For this review, take the finished solid that the model builds, in its own axes (mm). A direction names the side the tool comes from. Give positions to 0.01 mm unless a question says otherwise; leave off trailing zeros. Loops run counter-clockwise (first coordinate to the right, second up) from the corner with the lowest first, then second, coordinate; pieces in that order, holes last. Notation, with made-up numbers: (59, 2.5) - (74, 2.5) arc R18 cw to (74, 9.5) - close; hole circle Ø3 at (0.25, 31.5). An arc over 180 degrees is marked (long way). Put each result on its own line as item: value.
Autodesk Inventor part; units mm, degrees
ref_plane "YZ Plane" through (0, 0, 0) normal (1, 0, 0) x (0, 1, 0)
ref_plane "XZ Plane" through (0, 0, 0) normal (0, 1, 0) x (-1, 0, 0)
ref_plane "XY Plane" through (0, 0, 0) normal (0, 0, 1) x (1, 0, 0)
ref_plane "Work Plane1" through (0, 0, 0) normal (0, 0, 1) x (1, 0, 0)
sketch "Sketch1" plane through (0, 0, 0) normal (0, 0, 1) x (1, 0, 0)
  arc A0 (-3.651, 13.5937) -> (-4.7619, 15.391) centre (-4.2064, 14.4923) ccw
  arc A1 (-3.651, 13.5937) -> (-6.4477, 10.2643) centre (0, 7.6875) ccw
  arc A2 (-8.4097, 11.0483) -> (-6.4477, 10.2643) centre (-7.4287, 10.6563) ccw
  arc A3 (-4.7619, 15.391) -> (-8.4097, 11.0483) centre (0, 7.6875) ccw
  arc A4 (6.4477, 10.2643) -> (8.4097, 11.0483) centre (7.4287, 10.6563) ccw
  arc A5 (6.4477, 10.2643) -> (3.651, 13.5937) centre (0, 7.6875) ccw
  arc A6 (4.7619, 15.391) -> (3.651, 13.5937) centre (4.2064, 14.4923) ccw
  arc A7 (8.4097, 11.0483) -> (4.7619, 15.391) centre (0, 7.6875) ccw
  arc A8 (-6.4563, 5.1322) -> (-8.4209, 4.3547) centre (-7.4386, 4.7434) ccw
  arc A9 (-6.4563, 5.1322) -> (-3.651, 1.7813) centre (0, 7.6875) ccw
  arc A10 (-4.7619, -0.016) -> (-3.651, 1.7813) centre (-4.2064, 0.8827) ccw
  arc A11 (-8.4209, 4.3547) -> (-4.7619, -0.016) centre (0, 7.6875) ccw
  arc A12 (3.651, 1.7813) -> (4.7619, -0.016) centre (4.2064, 0.8827) ccw
  arc A13 (3.651, 1.7813) -> (6.4563, 5.1322) centre (0, 7.6875) ccw
  arc A14 (8.4209, 4.3547) -> (6.4563, 5.1322) centre (7.4386, 4.7434) ccw
  arc A15 (4.7619, -0.016) -> (8.4209, 4.3547) centre (0, 7.6875) ccw
  circle A16 centre (10.65, 7.6999) radius 1.15
  circle A17 centre (0, 15.6875) radius 1.0564
  circle A18 centre (0, -0.3125) radius 1.0564
  circle A19 centre (0, 7.6875) radius 5
  circle A20 centre (0, 7.6875) radius 13.7
  line L0 (-116.625, -11.1875) -> (15.375, -11.1875)
  line L1 (15.375, -11.1875) -> (15.375, -7.6875)
  line L2 (-116.625, -7.6875) -> (15.375, -7.6875)
  line L3 (-116.625, -11.1875) -> (-116.625, -7.6875)
  line L4 (15.375, -7.6875) -> (-15.375, -7.6875)
  line L5 (-15.375, -7.6875) -> (-15.375, 22.3125)
  line L6 (-15.375, 22.3125) -> (15.375, 22.3125)
  line L7 (15.375, 22.3125) -> (15.375, -7.6875)
  circle A21 centre (0, 7.6875) radius 14.375
  circle A22 centre (0, 7.6875) radius 5.2
  arc A23 (-3.4406, 13.2535) -> (-4.9722, 15.7312) centre (-4.2064, 14.4923) ccw
  arc A24 (-3.4406, 13.2535) -> (-6.0763, 10.1158) centre (0, 7.6875) ccw
  arc A25 (-8.7812, 11.1968) -> (-6.0763, 10.1158) centre (-7.4287, 10.6563) ccw
  arc A26 (-4.9722, 15.7312) -> (-8.7812, 11.1968) centre (0, 7.6875) ccw
  arc A27 (4.9722, 15.7312) -> (3.4406, 13.2535) centre (4.2064, 14.4923) ccw
  arc A28 (6.0763, 10.1158) -> (3.4406, 13.2535) centre (0, 7.6875) ccw
  arc A29 (6.0763, 10.1158) -> (8.7812, 11.1968) centre (7.4287, 10.6563) ccw
  arc A30 (8.7812, 11.1968) -> (4.9722, 15.7312) centre (0, 7.6875) ccw
  arc A31 (3.4406, 2.1215) -> (6.0844, 5.2794) centre (0, 7.6875) ccw
  arc A32 (3.4406, 2.1215) -> (4.9722, -0.3562) centre (4.2064, 0.8827) ccw
  arc A33 (4.9722, -0.3562) -> (8.7928, 4.2075) centre (0, 7.6875) ccw
  arc A34 (8.7928, 4.2075) -> (6.0844, 5.2794) centre (7.4386, 4.7434) ccw
  arc A35 (-6.0844, 5.2794) -> (-8.7928, 4.2075) centre (-7.4386, 4.7434) ccw
  arc A36 (-6.0844, 5.2794) -> (-3.4406, 2.1215) centre (0, 7.6875) ccw
  arc A37 (-4.9722, -0.3562) -> (-3.4406, 2.1215) centre (-4.2064, 0.8827) ccw
  arc A38 (-8.7928, 4.2075) -> (-4.9722, -0.3562) centre (0, 7.6875) ccw
  circle A39 centre (10.65, 7.6999) radius 1.55
  point P0 (0, 0)
  dimension "d0" = 30
  dimension "d1" = 15.375
  dimension "d2" = 15.375
  dimension "d3" = 0.2
  dimension "d4" = 0.4
  dimension "d5" = 0.4
  dimension "d6" = 0.4
  dimension "d7" = 0.4
  dimension "d8" = 0.4
extrude "Extrusion1" add sketch "Sketch1" along normal blind 1 contours A20 | L2 L5 L6 L7 | A21
sketch "Sketch2" plane through (0, 0, 1) normal (0, 0, 1) x (1, 0, 0)
  line L0 (15.375, 22.3125) -> (-15.375, 22.3125)
  line L1 (-15.375, 22.3125) -> (-15.375, -7.6875)
  line L2 (-15.375, -7.6875) -> (15.375, -7.6875)
  line L3 (15.375, -7.6875) -> (15.375, 22.3125)
  circle A0 centre (0, 15.6875) radius 1.0564
  circle A1 centre (0, -0.3125) radius 1.0564
  circle A2 centre (0, 7.6875) radius 5.2
  arc A3 (-3.4406, 13.2535) -> (-6.0763, 10.1158) centre (0, 7.6875) ccw
  arc A4 (-8.7812, 11.1968) -> (-6.0763, 10.1158) centre (-7.4287, 10.6563) ccw
  arc A5 (-4.9722, 15.7312) -> (-8.7812, 11.1968) centre (0, 7.6875) ccw
  arc A6 (-3.4406, 13.2535) -> (-4.9722, 15.7312) centre (-4.2064, 14.4923) ccw
  arc A7 (6.0763, 10.1158) -> (3.4406, 13.2535) centre (0, 7.6875) ccw
  arc A8 (4.9722, 15.7312) -> (3.4406, 13.2535) centre (4.2064, 14.4923) ccw
  arc A9 (8.7812, 11.1968) -> (4.9722, 15.7312) centre (0, 7.6875) ccw
  arc A10 (6.0763, 10.1158) -> (8.7812, 11.1968) centre (7.4287, 10.6563) ccw
  arc A11 (3.4406, 2.1215) -> (4.9722, -0.3562) centre (4.2064, 0.8827) ccw
  arc A12 (3.4406, 2.1215) -> (6.0844, 5.2794) centre (0, 7.6875) ccw
  arc A13 (8.7928, 4.2075) -> (6.0844, 5.2794) centre (7.4386, 4.7434) ccw
  arc A14 (4.9722, -0.3562) -> (8.7928, 4.2075) centre (0, 7.6875) ccw
  arc A15 (-6.0844, 5.2794) -> (-3.4406, 2.1215) centre (0, 7.6875) ccw
  arc A16 (-4.9722, -0.3562) -> (-3.4406, 2.1215) centre (-4.2064, 0.8827) ccw
  arc A17 (-8.7928, 4.2075) -> (-4.9722, -0.3562) centre (0, 7.6875) ccw
  arc A18 (-6.0844, 5.2794) -> (-8.7928, 4.2075) centre (-7.4386, 4.7434) ccw
  circle A19 centre (10.65, 7.6999) radius 1.55
  arc A20 (4.9722, 15.7312) -> (3.4406, 13.2535) centre (4.2064, 14.4923) ccw
  line L4 (4.2064, 15.9488) -> (15.375, 15.9488)
  line L5 (15.375, -7.6875) -> (15.375, 22.3125)
  line L6 (4.2064, -0.5738) -> (15.375, -0.5738)
  arc A21 (6.0763, 10.1158) -> (8.7812, 11.1968) centre (7.4287, 10.6563) ccw
  line L7 (6.0763, 10.1158) -> (6.0844, 5.2794)
  point P0 (0, 0)
extrude "Extrusion2" add sketch "Sketch2" along normal blind 1.5 contours L3 L4 A8 A7 L7 A12 A11 L6 L2 L1 L0
sketch "Sketch3" plane through (0, 0, 2.5) normal (0, 0, 1) x (1, 0, 0)
  line L0 (15.375, -7.6875) -> (15.375, -0.5738)
  line L1 (15.375, -0.5738) -> (4.2064, -0.5738)
  arc A0 (3.4406, 2.1215) -> (4.2064, -0.5738) centre (4.2064, 0.8827) ccw
  arc A1 (3.4406, 2.1215) -> (6.0844, 5.2794) centre (0, 7.6875) ccw
  line L2 (6.0844, 5.2794) -> (6.0763, 10.1158)
  arc A2 (6.0763, 10.1158) -> (3.4406, 13.2535) centre (0, 7.6875) ccw
  arc A3 (4.2064, 15.9488) -> (3.4406, 13.2535) centre (4.2064, 14.4923) ccw
  line L3 (4.2064, 15.9488) -> (15.375, 15.9488)
  line L4 (15.375, 15.9488) -> (15.375, 22.3125)
  line L5 (15.375, 22.3125) -> (-15.375, 22.3125)
  line L6 (-15.375, 22.3125) -> (-15.375, -7.6875)
  line L7 (-15.375, -7.6875) -> (15.375, -7.6875)
  circle A4 centre (0, 15.6875) radius 1.0564
  circle A5 centre (0, -0.3125) radius 1.0564
  arc A6 (-6.0844, 5.2794) -> (-8.7928, 4.2075) centre (-7.4386, 4.7434) ccw
  arc A7 (-6.0844, 5.2794) -> (-3.4406, 2.1215) centre (0, 7.6875) ccw
  arc A8 (-4.9722, -0.3562) -> (-3.4406, 2.1215) centre (-4.2064, 0.8827) ccw
  arc A9 (-8.7928, 4.2075) -> (-4.9722, -0.3562) centre (0, 7.6875) ccw
  arc A10 (-3.4406, 13.2535) -> (-4.9722, 15.7312) centre (-4.2064, 14.4923) ccw
  arc A11 (-3.4406, 13.2535) -> (-6.0763, 10.1158) centre (0, 7.6875) ccw
  arc A12 (-8.7812, 11.1968) -> (-6.0763, 10.1158) centre (-7.4287, 10.6563) ccw
  arc A13 (-4.9722, 15.7312) -> (-8.7812, 11.1968) centre (0, 7.6875) ccw
  circle A14 centre (0, 7.6875) radius 5.2
  circle A15 centre (0, 15.6875) radius 2.65
  circle A16 centre (0, -0.3125) radius 1.0564
  circle A17 centre (0, -0.3125) radius 2.65
  arc A18 (-2.4425, 10.6818) -> (-4.3563, 11.5819) centre (-5.3868, 6.906) ccw
  arc A19 (-4.3563, 11.5819) -> (-4.9119, 10.8525) centre (0, 7.6875) ccw
  arc A20 (-4.9119, 10.8525) -> (-3.5356, 9.2466) centre (-0.678, 13.0883) ccw
  arc A21 (-3.5356, 9.2466) -> (-3.736, 8.6743) centre (0, 7.6875) ccw
  arc A22 (-3.736, 8.6743) -> (-5.8134, 8.2775) centre (-3.8987, 3.889) ccw
  arc A23 (-5.8134, 8.2775) -> (-5.8341, 7.3609) centre (0, 7.6875) ccw
  arc A24 (-5.8341, 7.3609) -> (-3.7768, 6.8706) centre (-3.723, 11.6584) ccw
  arc A25 (-3.7768, 6.8706) -> (-3.6025, 6.2899) centre (0, 7.6875) ccw
  arc A26 (-3.6025, 6.2899) -> (-5.05, 4.7478) centre (-0.9214, 2.3228) ccw
  arc A27 (-5.05, 4.7478) -> (-4.5279, 3.994) centre (0, 7.6875) ccw
  arc A28 (-4.5279, 3.994) -> (-2.5753, 4.8067) centre (-5.346, 8.7117) ccw
  arc A29 (-2.5753, 4.8067) -> (-2.093, 4.4393) centre (0, 7.6875) ccw
  arc A30 (-2.093, 4.4393) -> (-2.3576, 2.341) centre (2.4078, 2.8058) ccw
  arc A31 (-2.3576, 2.341) -> (-1.4922, 2.038) centre (0, 7.6875) ccw
  arc A32 (-1.4922, 2.038) -> (-0.3902, 3.8431) centre (-4.927, 5.3738) ccw
  arc A33 (-0.3902, 3.8431) -> (0.216, 3.8294) centre (0, 7.6875) ccw
  arc A34 (0.216, 3.8294) -> (1.2353, 1.9763) centre (4.8174, 5.1534) ccw
  arc A35 (1.2353, 1.9763) -> (2.1135, 2.2398) centre (0, 7.6875) ccw
  arc A36 (2.1135, 2.2398) -> (1.944, 4.348) centre (-2.6261, 2.9196) ccw
  arc A37 (1.944, 4.348) -> (2.4425, 4.6932) centre (0, 7.6875) ccw
  arc A38 (2.4425, 4.6932) -> (4.3563, 3.7931) centre (5.3868, 8.469) ccw
  arc A39 (4.3563, 3.7931) -> (4.9119, 4.5225) centre (0, 7.6875) ccw
  arc A40 (4.9119, 4.5225) -> (3.5356, 6.1284) centre (0.678, 2.2867) ccw
  arc A41 (3.5356, 6.1284) -> (3.736, 6.7007) centre (0, 7.6875) ccw
  arc A42 (3.736, 6.7007) -> (5.8134, 7.0975) centre (3.8987, 11.486) ccw
  arc A43 (5.8134, 7.0975) -> (5.8341, 8.0141) centre (0, 7.6875) ccw
  arc A44 (5.8341, 8.0141) -> (3.7768, 8.5044) centre (3.723, 3.7166) ccw
  arc A45 (3.7768, 8.5044) -> (3.6025, 9.0851) centre (0, 7.6875) ccw
  arc A46 (3.6025, 9.0851) -> (5.05, 10.6272) centre (0.9214, 13.0522) ccw
  arc A47 (5.05, 10.6272) -> (4.5279, 11.381) centre (0, 7.6875) ccw
  arc A48 (4.5279, 11.381) -> (2.5753, 10.5683) centre (5.346, 6.6633) ccw
  arc A49 (2.5753, 10.5683) -> (2.093, 10.9357) centre (0, 7.6875) ccw
  arc A50 (2.093, 10.9357) -> (2.3576, 13.034) centre (-2.4078, 12.5692) ccw
  arc A51 (2.3576, 13.034) -> (1.4922, 13.337) centre (0, 7.6875) ccw
  arc A52 (1.4922, 13.337) -> (0.3902, 11.5319) centre (4.927, 10.0012) ccw
  arc A53 (0.3902, 11.5319) -> (-0.216, 11.5456) centre (0, 7.6875) ccw
  arc A54 (-0.216, 11.5456) -> (-1.2353, 13.3987) centre (-4.8174, 10.2216) ccw
  arc A55 (-1.2353, 13.3987) -> (-2.1135, 13.1352) centre (0, 7.6875) ccw
  arc A56 (-2.1135, 13.1352) -> (-1.944, 11.027) centre (2.6261, 12.4554) ccw
  arc A57 (-1.944, 11.027) -> (-2.4425, 10.6818) centre (0, 7.6875) ccw
  circle A58 centre (0, 7.6875) radius 5.8433
  circle A59 centre (0, 7.6875) radius 6.5436
  arc A60 (-3.4406, 13.2535) -> (-4.9722, 15.7312) centre (-4.2064, 14.4923) ccw
  line L8 (-2.9676, 15.2581) -> (-2.615, 15.2581)
  arc A61 (4.9722, 15.7312) -> (3.4406, 13.2535) centre (4.2064, 14.4923) ccw
  line L9 (2.9676, 15.2581) -> (2.615, 15.2581)
  arc A62 (3.4406, 2.1215) -> (4.9722, -0.3562) centre (4.2064, 0.8827) ccw
  line L10 (2.8055, 0.4846) -> (2.5273, 0.4846)
  arc A63 (-4.9722, -0.3562) -> (-3.4406, 2.1215) centre (-4.2064, 0.8827) ccw
  line L11 (-2.8055, 0.4846) -> (-2.5273, 0.4846)
  arc A64 (-8.7812, 11.1968) -> (-6.0763, 10.1158) centre (-7.4287, 10.6563) ccw
  line L12 (-7.7556, 9.237) -> (-7.7556, 6.165)
  point P0 (0, 0)
  point P1 (-6.0844, 5.2794)
  point P2 (-6.0763, 10.1158)
  point P3 (2.9676, 15.2581)
  dimension "d13" = 5.3
  dimension "d14" = 5.3
extrude "Extrusion3" add sketch "Sketch3" along normal blind 1 contours L7 L6 L5 L4 L3 A3 L9 A15 L8 A10 A13 A12 L12 A6 A9 A8 L11 A17 L10 A0 L1 L0
sketch "Sketch4" plane through (0, 0, 3.5) normal (0, 0, 1) x (1, 0, 0)
  line L0 (15.375, -0.5738) -> (4.2064, -0.5738)
  arc A0 (2.8055, 0.4846) -> (4.2064, -0.5738) centre (4.2064, 0.8827) ccw
  line L1 (2.8055, 0.4846) -> (2.5273, 0.4846)
  arc A1 (-2.5273, 0.4846) -> (2.5273, 0.4846) centre (0, -0.3125) ccw
  line L2 (-2.5273, 0.4846) -> (-2.8055, 0.4846)
  arc A2 (-4.9722, -0.3562) -> (-2.8055, 0.4846) centre (-4.2064, 0.8827) ccw
  arc A3 (-8.7928, 4.2075) -> (-4.9722, -0.3562) centre (0, 7.6875) ccw
  arc A4 (-7.7556, 6.165) -> (-8.7928, 4.2075) centre (-7.4386, 4.7434) ccw
  line L3 (-7.7556, 6.165) -> (-7.7556, 9.237)
  arc A5 (-8.7812, 11.1968) -> (-7.7556, 9.237) centre (-7.4287, 10.6563) ccw
  arc A6 (-4.9722, 15.7312) -> (-8.7812, 11.1968) centre (0, 7.6875) ccw
  arc A7 (-2.9676, 15.2581) -> (-4.9722, 15.7312) centre (-4.2064, 14.4923) ccw
  line L4 (-2.9676, 15.2581) -> (-2.615, 15.2581)
  arc A8 (2.615, 15.2581) -> (-2.615, 15.2581) centre (0, 15.6875) ccw
  line L5 (2.615, 15.2581) -> (2.9676, 15.2581)
  arc A9 (4.2064, 15.9488) -> (2.9676, 15.2581) centre (4.2064, 14.4923) ccw
  line L6 (4.2064, 15.9488) -> (15.375, 15.9488)
  line L7 (15.375, 15.9488) -> (15.375, 22.3125)
  line L8 (15.375, 22.3125) -> (-15.375, 22.3125)
  line L9 (-15.375, 22.3125) -> (-15.375, -7.6875)
  line L10 (-15.375, -7.6875) -> (15.375, -7.6875)
  line L11 (15.375, -7.6875) -> (15.375, -0.5738)
  circle A10 centre (-12.125, -4.4375) radius 3.25
  circle A11 centre (12.125, -4.4375) radius 3.25
  point P0 (0, 0)
  dimension "d17" = 6.5
  dimension "d18" = 6.5
hole "Hole1" at (-12.125, -4.4375, 3.5) at (12.125, -4.4375, 3.5) direction (0, 0, -1) diameter 3.6 end through all
equation "\"d2\" = d1"
properties part number "front_motur_holder"
1) Take a section at D-D on z = 1.65. State the section outline as (x, y) points (1 decimal), and give its area (3 significant figures).
Geometry check:
outline: (-15.4, -7.7) - (15.4, -7.7) - (15.4, -0.6) - (4.2, -0.6) arc R1.5 cw to (3.4, 2.1) arc R6.5 ccw to (6.1, 5.3) - (6.1, 10.1) arc R6.5 ccw to (3.4, 13.3) arc R1.5 cw to (4.2, 15.9) - (15.4, 15.9) - (15.4, 22.3) - (-15.4, 22.3) - close; hole circle Ø3.6 at (-12.1, -4.4); hole (-8.8, 4.2) arc R9.5 ccw to (-5, -0.4) arc R1.5 ccw to (-3.4, 2.1) arc R6.5 cw to (-6.1, 5.3) arc R1.5 ccw to start; hole (-8.8, 11.2) arc R1.5 ccw to (-6.1, 10.1) arc R6.5 cw to (-3.4, 13.3) arc R1.5 ccw to (-5, 15.7) arc R9.5 ccw to start; hole circle Ø10.4 at (0, 7.7); hole circle Ø2.1 at (0, -0.3); hole circle Ø2.1 at (0, 15.7); hole circle Ø3.6 at (12.1, -4.4)
area: 590 mm²
2) Take a section at C-C on x = 7.5. State the section outline as (y, z) points, and give its area (3 significant figures).
Geometry check:
outline: (-7.69, 0) - (1.93, 0) - (1.93, 1) - (-0.57, 1) - (-0.57, 3.5) - (-7.69, 3.5) - close; (6.2, 0) - (9.2, 0) - (9.2, 1) - (6.2, 1) - close; (13.45, 0) - (22.31, 0) - (22.31, 3.5) - (15.95, 3.5) - (15.95, 1) - (13.45, 1) - close
area: 55.2 mm²
3) For faces 4 (the face through (3.34, -0.29, 2.99)), 5 (the face through (0.07, -2.96, 2.99)), 6 (the face through (5.036, 3.51, 1.232)), 7 (the face through (-7.756, 8, 3)), list the 3-axis set-ups (+Z, -Z, +X, -X, +Y, -Y) from which the entire face can be reached by the end or side of a thin tool; tool diameter is ignored.
Geometry check:
face 4: +Z, -Z, +X
face 5: +Z
face 6: +Z, -Z
face 7: +Z, +X
4) Wall thickness on line 1 (Y direction, x = 0, z = 0.6); line 2 (Y direction, x = 8.5, z = 1.8); line 3 (X direction, y = 4.25, z = 2.1) (3 decimals): over which ranges is each line inside the solid? List them lowest first.
Geometry check:
line 1: y = -7.69 to -1.37, 0.74 to 2.49, 12.89 to 14.63, 16.74 to 22.31
line 2: y = -7.69 to -0.57, 15.95 to 22.31
line 3: x = -15.375 to -8.809, -5.568 to -3.902, 3.902 to 5.568
5) Draft analysis for pull direction Y (two halves, no side actions). For faces 1 (the face through (-5.03, 11.87, 1.23)), 2 (the face through (-10, 8, 3.5)), 3 (the face through (7.214, 13.802, 0.493)), state which applies: pulls with the +Y half, pulls with the -Y half, needs draft (parallel to the pull), parting line crosses it, or undercut.
Geometry check:
face 1: undercut
face 2: needs draft
face 3: undercut
6) Take a section at A-A on x = -4. State the section outline as (y, z) points.
Geometry check:
outline: (-7.69, 0) - (-0.56, 0) - (-0.56, 3.5) - (-7.69, 3.5) - close; (2.51, 0) - (4.36, 0) - (4.36, 2.5) - (2.51, 2.5) - close; (11.01, 0) - (12.87, 0) - (12.87, 2.5) - (11.01, 2.5) - close; (15.93, 0) - (22.31, 0) - (22.31, 3.5) - (15.93, 3.5) - close
7) Take a section at B-B on y = 14.25. State the section outline as (x, z) points (3 decimals).
Geometry check:
outline: (-15.375, 0) - (-6.809, 0) - (-6.809, 3.5) - (-15.375, 3.5) - close; (-2.77, 0) - (2.77, 0) - (2.77, 2.5) - (-2.77, 2.5) - close; (6.809, 0) - (15.375, 0) - (15.375, 1) - (6.809, 1) - close
8) Insertion check: pin 1 Ø1.1 at (y, z) = (7, 3) entering from +X; pin 2 Ø11 at (x, y) = (-2, 9) entering from +Z; pin 3 Ø5.5 at (x, y) = (9.5, 8) entering from +Z. Each pin has a flat end and moves straight along its axis. Give the tip position at first contact, or say it passes through.
Geometry check:
pin 1: stops at x = 6.08
pin 2: stops at z = 2.5
pin 3: stops at z = 1
